Could you check a few things on this model? Use its own coordinates, in mm. A direction names the side the tool comes from. Coordinates: 2 decimals unless noted, no trailing zeros. Order: outer loops, then holes, each group sorted by start corner. A loop starts at its lowest first (then second) coordinate and runs counter-clockwise, first axis right, second up. Notation, with made-up numbers: (-22.75, 18.5) -> (-6.75, 18.5) arc R22 ccw to (-6.75, 38.5) -> close; hole circle Ø10 at (-13, 3.5). An arc over 180 degrees is marked (long way). Put each result on its own line as item: value. Start each with the question number.
Q1. If we section it at C-C (y = 16.5): Please give me the cut outline in (x, z).
Q2. If we section it at B-B (z = 5.5): Please give me the cut outline in (x, y).
Q3. If we section it at A-A (x = 0): Please give me the cut outline in (y, z).
Q4. If we section it at D-D (z = 12.7): Please give me the cut outline in (x, y).
Q5. Will these pins go through, and if not, where does the flat tip stop? pin 1 (4 mm diameter, centred on y = -12.5, z = 22.5, fed in from +X); pin 2 (6 mm diameter, centred on y = -19, z = 3.5, fed in from +X); pin 3 (8 mm diameter, centred on x = 3.5, y = -10.5, fed in from -Z); pin 4 (3.5 mm diameter, centred on x = 1, z = 12, fed in from -Y).
Q6. For faces 1 (the face through (0.73, 16.01, 9.4)), 2 (the face through (-5.525, 3.131, 12.878)), which set-ups out of +Z, -Z, +X, -X, +Y, -Y let a thin tool reach every point of the face, with its end or its side?
Q7. Please list where these lines run through material, in increasing order: line 1 along Z through (x, y) = (0, -18.5); line 2 along X through (y, z) = (-8, 12); line 3 along Y through (x, z) = (6, 23.25).
Q8. We'd pull the mould along X, two halves only. Please class faces 3 (the face through (5.474, 3.219, 12.878)), 4 (the face through (5, -5, 25.4)), 5 (the face through (-5.506, 24.796, 12.522)): +X half, -X half, draft (parallel to the pull), parting line (faces both ways), or undercut.
Autodesk Inventor part; units mm, degrees
ref_plane "YZ Plane" through (0, 0, 0) normal (1, 0, 0) x (0, 1, 0)
ref_plane "XY Plane" through (0, 0, 0) normal (0, 0, 1) x (1, 0, 0)
sketch "Sketch1" plane through (0, 0, 0) normal (0, 0, 1) x (1, 0, 0)
  circle A0 centre (0, 0) radius 25.4
  dimension "d0" = 50.8
extrude "Extrusion1" add sketch "Sketch1" along normal blind 25.4
ref_plane "Work Plane1" through (0, 25.4, 0) normal (0, 1, 0) x (-1, 0, 0)
sketch "Sketch2" plane through (0, 25.4, 0) normal (0, 1, 0) x (-1, 0, 0)
  line L0 (0, 0) -> (0, 12.7)
  circle A0 centre (0, 12.7) radius 3.3782
  dimension "d3" = 12.7
  dimension "d4" = 6.7564
extrude "Extrusion2" cut sketch "Sketch2" against normal blind 50.8
sketch "Sketch3" plane through (0, 0, 25.4) normal (0, 0, 1) x (1, 0, 0)
  circle A0 centre (0, 0) radius 25.4
  circle A1 centre (0, 0) radius 6.35
  line L0 (3.6662, 6.35) -> (7.3323, 0)
  line L1 (7.3323, 0) -> (3.6662, -6.35)
  line L2 (3.6662, -6.35) -> (-3.6662, -6.35)
  line L3 (-3.6662, -6.35) -> (-7.3323, 0)
  line L4 (-7.3323, 0) -> (-3.6662, 6.35)
  line L5 (-3.6662, 6.35) -> (3.6662, 6.35)
  point P0 (0, 6.35)
  dimension "d7" = 12.7
extrude "Extrusion3" cut sketch "Sketch3" against normal blind 50.8 contours A1 | A1 L0 L1 | A1 L5 L0 | L1 L2 A1 | A1 L4 L5 | L2 L3 A1 | A1 L3 L4
properties part number "insert" material "Aluminum 6061"
The answers:
1. outline: (-19.31, 0) -> (19.31, 0) -> (19.31, 25.4) -> (-19.31, 25.4) -> close; hole circle Ø6.76 at (0, 12.7)
2. outline: circle Ø50.8 at (0, 0); hole (-7.33, 0) -> (-3.67, -6.35) -> (3.67, -6.35) -> (7.33, 0) -> (3.67, 6.35) -> (-3.67, 6.35) -> close
3. outline: (-25.4, 0) -> (-6.35, 0) -> (-6.35, 9.32) -> (-25.4, 9.32) -> close; (-25.4, 16.08) -> (-6.35, 16.08) -> (-6.35, 25.4) -> (-25.4, 25.4) -> close; (6.35, 0) -> (25.4, 0) -> (25.4, 9.32) -> (6.35, 9.32) -> close; (6.35, 16.08) -> (25.4, 16.08) -> (25.4, 25.4) -> (6.35, 25.4) -> close
4. outline: (-7.33, 0) -> (-3.67, 6.35) -> (-3.38, 6.35) -> (-3.38, 25.17) arc R25.4 ccw to (-3.38, -25.17) -> (-3.38, -6.35) -> (-3.67, -6.35) -> close; (3.38, -25.17) arc R25.4 ccw to (3.38, 25.17) -> (3.38, 6.35) -> (3.67, 6.35) -> (7.33, 0) -> (3.67, -6.35) -> (3.38, -6.35) -> close
5. pin 1: x = 23.13
5. pin 2: x = 19.73
5. pin 3: z = 0
5. pin 4: through
6. face 1: +Y, -Y
6. face 2: +Z, -Z
7. line 1: 0 to 9.32, 16.08 to 25.4
7. line 2: -24.11 to -3.3, 3.3 to 24.11
7. line 3: -24.68 to -2.31, 2.31 to 24.68
8. face 3: undercut
8. face 4: draft
8. face 5: parting line
